The figure shows three views and two pictorial views of one solid part (mm, origin at its lowest corner). Answer the questions. Coordinates: 2 decimals unless noted, no trailing zeros. Order: outer loops, then holes, each group sorted by start corner. A loop starts at its lowest first (then second) coordinate and runs counter-clockwise, first axis right, second up. Notation, with made-up numbers: M 82,67 L 96,67 A16 ccw 96,79 Z; hole C 17,41 d10. An arc over 180 degrees is marked long. Use a Markdown table: item, result.
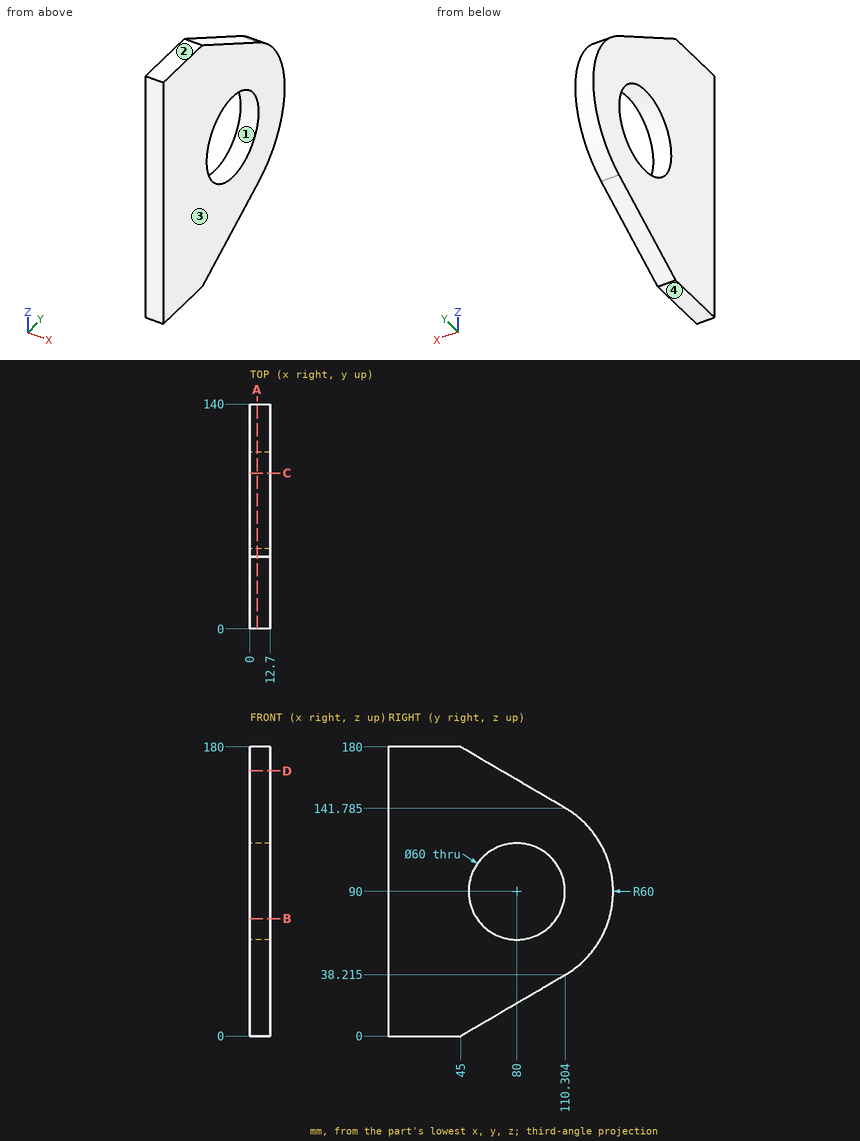
1. Find the intervals of material crossed by probe 1 along Y at (x, z) = (5.5, 90); probe 2 along Z at (x, y) = (10.5, 75); probe 3 along Z at (x, y) = (2, 56), in increasing order.
Answers below:
| item | result |
|---|---|
| probe 1 | 0 to 50, 110 to 140 |
| probe 2 | 17.56 to 60.42, 119.58 to 162.44 |
| probe 3 | 6.44 to 72, 108 to 173.56 |
2. Section B-B on z = 73 is taken. Determine the outline of the cut face in (x, y).
Answers below:
| item | result |
|---|---|
| outline | M 0,0 L 12.7,0 L 12.7,55.28 L 0,55.28 Z; M 0,104.72 L 12.7,104.72 L 12.7,137.54 L 0,137.54 Z |
3. For a pull along Z with two mould halves and no side action, classify the marked faces 1, 2, 3 and 4 as +Z half, -Z half, draft (parallel to the pull), parting line (faces both ways), or undercut.
Answers below:
| item | result |
|---|---|
| face 1 | undercut |
| face 2 | +Z half |
| face 3 | draft |
| face 4 | -Z half |
4. Flat-ended cylindrical pins translate along their axes: P1, Ø6, axis at x = 8, y = 62, coming from the -Z side; P2, Ø1, axis at x = 4.5, z = 73.5, coming from the +Y side; P3, Ø1.5, axis at x = 5.5, y = 81.5, coming from the -Z side. Find the tip coordinate at first contact, or state that the pin passes through.
Answers below:
| item | result |
|---|---|
| P1 | z = 8.19 |
| P2 | y = 137.83 |
| P3 | z = 20.92 |
5. Section D-D on z = 165 is taken. Determine the outline of the cut face in (x, y).
Answers below:
| item | result |
|---|---|
| outline | M 0,0 L 12.7,0 L 12.7,70.63 L 0,70.63 Z |
6. Section A-A on x = 4.5 is taken. Determine the outline of the cut face in (y, z) (3 decimals), then the cut area to 3 significant figures.
Answers below:
| item | result |
|---|---|
| outline | M 0,0 L 45,0 L 110.304,38.215 A60 ccw 110.304,141.785 L 45,180 L 0,180 Z; hole C 80,90 d60 |
| area | 16,700 mm² |
7. Section C-C on y = 97 is taken. Determine the outline of the cut face in (x, z), then the cut area to 3 significant figures.
Answers below:
| item | result |
|---|---|
| outline | M 0,30.43 L 12.7,30.43 L 12.7,65.28 L 0,65.28 Z; M 0,114.72 L 12.7,114.72 L 12.7,149.57 L 0,149.57 Z |
| area | 885 mm² |
